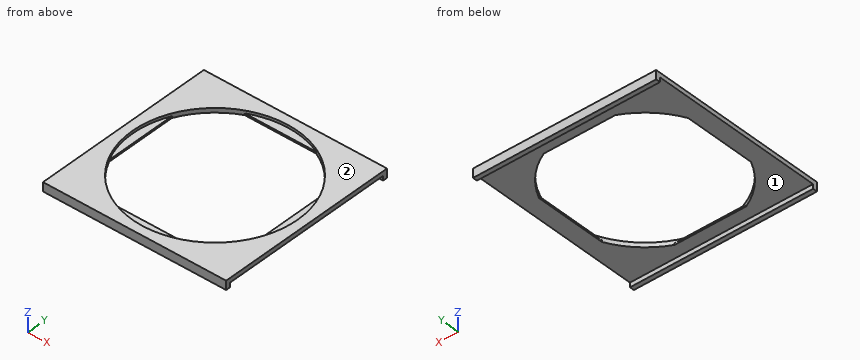
from build123d import *

# Parameters (mm, degrees)
SKETCH_7_W               = 400
SKETCH_7_H               = 400
EXTRUDE_1_DEPTH          = 3
SKETCH_8_W               = 380
SKETCH_8_H               = 2
EXTRUDE_2_DEPTH          = 140
SKETCH_9_W               = 2
SKETCH_9_H               = 382
EXTRUDE_3_DEPTH          = 140
PATTERN_LINEAR_1_COUNT   = 12
PATTERN_LINEAR_1_PITCH   = 30
PATTERN_LINEAR_3_COUNT   = 12
PATTERN_LINEAR_3_PITCH   = 30
SKETCH_11_W              = 400
SKETCH_11_H              = 400
CUT_EXTRUDE_1_DEPTH      = 3
CUT_EXTRUDE_2_DEPTH      = 570.034269618
CUT_EXTRUDE_2_DEPTH_BACK = 570.034269618
SKETCH_12_R              = 300
SKETCH_12_R_2            = 90
SKETCH_13_R              = 92.5
SKETCH_13_R_2            = 89.5
EXTRUDE_8_DEPTH          = 140
SKETCH_14_W              = 205
SKETCH_14_H              = 205
SKETCH_14_W_2            = 185
SKETCH_14_H_2            = 185
EXTRUDE_9_DEPTH          = 5
EXTRUDE_10_DEPTH         = 2
PATTERN_CIRCULAR_1_COUNT = 4
CUT_EXTRUDE_START        = -140
SKETCH_16_R              = 92.5
CUT_EXTRUDE_3_DEPTH      = 140
SKETCH_17_W              = 205
SKETCH_17_H              = 5
EXTRUDE_11_DEPTH         = 5


with BuildPart() as part:
    # 草图7 → 凸台-拉伸1 (new body)
    with BuildSketch(Plane.XY):
        with Locations((200, 200)):
            Rectangle(SKETCH_7_W, SKETCH_7_H)
    extrude(amount=EXTRUDE_1_DEPTH)

    # 草图8 → 凸台-拉伸2 (add)
    with BuildSketch(Plane.XY.offset(3)):
        with Locations((200, 389)):
            Rectangle(SKETCH_8_W, SKETCH_8_H)
    extrude_2 = extrude(amount=EXTRUDE_2_DEPTH)

    # 草图9 → 凸台-拉伸3 (add)
    with BuildSketch(Plane.XY.offset(3)):
        with Locations((11, 199)):
            Rectangle(SKETCH_9_W, SKETCH_9_H)
    extrude_3 = extrude(amount=EXTRUDE_3_DEPTH)

    # 阵列(线性)1: 凸台-拉伸3 ×12
    with Locations(*[(i * PATTERN_LINEAR_1_PITCH, 0, 0) for i in range(1, PATTERN_LINEAR_1_COUNT)]):
        add(extrude_3)

    # 阵列(线性)3: 凸台-拉伸2 ×12
    with Locations(*[(0, -i * PATTERN_LINEAR_3_PITCH, 0) for i in range(1, PATTERN_LINEAR_3_COUNT)]):
        add(extrude_2)

    # 草图11 → 切除-拉伸1 (cut)
    with BuildSketch(Plane(origin=(0, 0, 0), x_dir=(-1, 0, 0), z_dir=(0, 0, -1))):
        with Locations((-200, 200)):
            Rectangle(SKETCH_11_W, SKETCH_11_H)
    extrude(amount=-CUT_EXTRUDE_1_DEPTH, mode=Mode.SUBTRACT)

    # 草图12 → 切除-拉伸2 (cut, two sides: drawn at the far end of the back side and taken through both)
    with BuildSketch(Plane(origin=(0, 0, 3), x_dir=(-1, 0, 0), z_dir=(0, 0, -1)).offset(-CUT_EXTRUDE_2_DEPTH_BACK)):
        with Locations((-191, 208.958405787)):
            Circle(SKETCH_12_R)
        with Locations((-191, 208.958405787)):
            Circle(SKETCH_12_R_2, mode=Mode.SUBTRACT)
    extrude(amount=CUT_EXTRUDE_2_DEPTH + CUT_EXTRUDE_2_DEPTH_BACK, mode=Mode.SUBTRACT)

    # 草图13 → 凸台-拉伸8 (add)
    with BuildSketch(Plane(origin=(0, 0, 3), x_dir=(-1, 0, 0), z_dir=(0, 0, -1))):
        with Locations((-191, 209)):
            Circle(SKETCH_13_R)
        with Locations((-191, 209)):
            Circle(SKETCH_13_R_2, mode=Mode.SUBTRACT)
    extrude(amount=-EXTRUDE_8_DEPTH)

    # 草图16 → 切除-拉伸3 (cut)
    with BuildSketch(Plane.XY.offset(143).offset(CUT_EXTRUDE_START)):
        with Locations(Location((191, 209, 0), (0, 0, 25.622027747))):
            Circle(SKETCH_16_R)
    extrude(amount=CUT_EXTRUDE_3_DEPTH, mode=Mode.SUBTRACT)


with BuildPart() as body_2:
    # 草图14 → 凸台-拉伸9 (new body)
    # profile 1 of 5: a face of its own
    with BuildSketch(Plane(origin=(0, 0, 3), x_dir=(-1, 0, 0), z_dir=(0, 0, -1))):
        with Locations((-191, 209)):
            Rectangle(SKETCH_14_W, SKETCH_14_H)
        with Locations((-191, 209)):
            Rectangle(SKETCH_14_W_2, SKETCH_14_H_2, mode=Mode.SUBTRACT)
    # profile 2 of 5: a face of its own
    with BuildSketch(Plane(origin=(0, 0, 3), x_dir=(-1, 0, 0), z_dir=(0, 0, -1))):
        with BuildLine():
            Line((-283.5, 209), (-283.5, 116.5))
            Line((-283.5, 116.5), (-191, 116.5))
            ThreePointArc((-191, 116.5), (-256.40737726, 143.59262274), (-283.5, 209))
        make_face()
    # profile 3 of 5: a face of its own
    with BuildSketch(Plane(origin=(0, 0, 3), x_dir=(-1, 0, 0), z_dir=(0, 0, -1))):
        with BuildLine():
            Line((-283.5, 301.5), (-283.5, 209))
            ThreePointArc((-283.5, 209), (-256.40737726, 274.40737726), (-191, 301.5))
            Line((-191, 301.5), (-283.5, 301.5))
        make_face()
    # profile 4 of 5: a face of its own
    with BuildSketch(Plane(origin=(0, 0, 3), x_dir=(-1, 0, 0), z_dir=(0, 0, -1))):
        with BuildLine():
            Line((-98.5, 301.5), (-191, 301.5))
            ThreePointArc((-191, 301.5), (-125.59262274, 274.40737726), (-98.5, 209))
            Line((-98.5, 209), (-98.5, 301.5))
        make_face()
    # profile 5 of 5: a face of its own
    with BuildSketch(Plane(origin=(0, 0, 3), x_dir=(-1, 0, 0), z_dir=(0, 0, -1))):
        with BuildLine():
            ThreePointArc((-98.5, 209), (-125.59262274, 143.59262274), (-191, 116.5))
            Line((-191, 116.5), (-98.5, 116.5))
            Line((-98.5, 116.5), (-98.5, 209))
        make_face()
    extrude(amount=EXTRUDE_9_DEPTH)

    # 草图15 → 凸台-拉伸10 (add)
    with BuildSketch(Plane(origin=(0, 0, -2), x_dir=(-1, 0, 0), z_dir=(0, 0, -1))):
        with BuildLine():
            Line((-231, 292.404136588), (-151, 292.404136588))
            ThreePointArc((-151, 292.404136588), (-191, 301.5), (-231, 292.404136588))
        make_face()
    extrude_10 = extrude(amount=-EXTRUDE_10_DEPTH)

    # 阵列(圆周)1: 凸台-拉伸10 ×4 about axis
    pattern_circular_1_axis = Axis((191, 209, 0), (0, 0, 1))
    for i in range(1, PATTERN_CIRCULAR_1_COUNT):
        add(extrude_10.rotate(pattern_circular_1_axis, i * 360 / PATTERN_CIRCULAR_1_COUNT))

    # 草图17 → 凸台-拉伸11 (add)
    with BuildSketch(Plane(origin=(0, 0, -2), x_dir=(-1, 0, 0), z_dir=(0, 0, -1))):
        with Locations((-191, 309)):
            Rectangle(SKETCH_17_W, SKETCH_17_H)
        with Locations((-191, 109)):
            Rectangle(SKETCH_17_W, SKETCH_17_H)
    extrude(amount=EXTRUDE_11_DEPTH)


solid = body_2.part
Read the model definition and answer for the solid it produces. Units are mm, in the model's axes. Face numbers are marked on the shaded views. Round coordinates to 2 decimals unless told otherwise and drop trailing zeros. Loops run counter-clockwise (first coordinate to the right, second up) from the corner with the lowest first, then second, coordinate; pieces in that order, holes last. Notation, with made-up numbers: (30, 48.5) - (88, 48.5) arc R26 ccw to (88, 85.5) - close; hole circle Ø11 at (80.25, -9.75). An arc over 180 degrees is marked (long way). One line per question, with ' | ' between items. Start each with the question number.
Q1. Section C-C on y = 175 is taken. Give the vertices of the cut face in (x, z), plus the area to 3 significant figures.
Q2. Section A-A on z = -5.5 is taken. Give the vertices of the cut face in (x, y).
Q3. Flat-ended cylindrical pins translate along their axes: pin 1 (4.5 mm diameter, centred on x = 279, y = 191.5, fed in from +Z); pin 2 (10 mm diameter, centred on x = 199.5, y = 297.5, fed in from +Z). Find the tip coordinate at first contact, or state that the pin passes through.
Q4. For a pull along Y with two mould halves and no side action, classify the marked faces 1 and 2 as +Y half, -Y half, draft (parallel to the pull), parting line (faces both ways), or undercut.
Q5. Find the intervals of material crossed by L1, parallel to Y at x = 150.5, z = -5.5; L2, parallel to X at y = 221, z = -1.5; L3, parallel to Y at x = 226, z = -1, in increasing order.
Q6. Section B-B on x = 172.5 is taken. Give the vertices of the cut face in (y, z).
Q7. Section D-D on x = 238 is taken. Give the vertices of the cut face in (y, z).
Established:
1) outline: (88.5, -2) - (107.6, -2) - (107.6, 0) - (104.98, 0) - (104.98, 3) - (88.5, 3) - close; (274.4, -2) - (293.5, -2) - (293.5, 3) - (277.02, 3) - (277.02, 0) - (274.4, 0) - close | area: 175 mm²
2) outline: (88.5, 106.5) - (293.5, 106.5) - (293.5, 111.5) - (88.5, 111.5) - close; (88.5, 306.5) - (293.5, 306.5) - (293.5, 311.5) - (88.5, 311.5) - close
3) pin 1: z = 0 | pin 2: z = 3
4) face 1: undercut | face 2: draft
5) L1: 106.5 to 111.5, 306.5 to 311.5 | L2: 88.5 to 107.6, 274.4 to 293.5 | L3: 106.5 to 125.6, 292.4 to 311.5
6) outline: (106.5, -7) - (111.5, -7) - (111.5, -2) - (125.6, -2) - (125.6, 0) - (118.37, 0) - (118.37, 3) - (106.5, 3) - close; (292.4, -2) - (306.5, -2) - (306.5, -7) - (311.5, -7) - (311.5, 3) - (299.63, 3) - (299.63, 0) - (292.4, 0) - close
7) outline: (106.5, -7) - (111.5, -7) - (111.5, -2) - (129.33, -2) - (129.33, 3) - (106.5, 3) - close; (288.67, -2) - (306.5, -2) - (306.5, -7) - (311.5, -7) - (311.5, 3) - (288.67, 3) - close
